For this review, take the finished solid that the model builds, in its own axes (mm). Face numbers are marked on the shaded views. A direction names the side the tool comes from. Round coordinates to 2 decimals unless told otherwise and drop trailing zeros. Write each loop counter-clockwise with the first axis right and the second up, starting at its lowest first coordinate (ties: lowest second). Pieces come first, ordered by that corner, then holes. Notation, with made-up numbers: M -18,-12.75 L -11,-12.75 A27 cw -11,19.25 Z; hole C 53,20 d9. An arc over 180 degrees is marked long. Write each question's results on one line, items separated by ' | '. Start each with the question number.
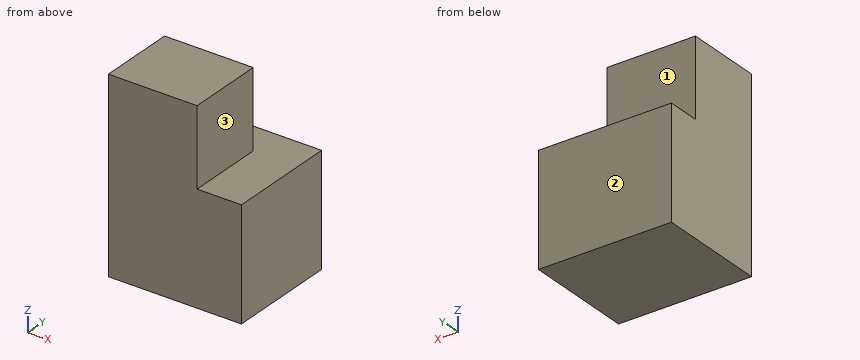
```python
from build123d import *

# Parameters (mm, degrees)
F1_W     = 40
F1_H     = 35
F3_DEPTH = 50
F2_W     = 40
F2_H     = 35
F4_DEPTH = 35


with BuildPart() as f3:
    # F1 (on Top) → F3 (new body)
    with BuildSketch(Plane.XY):
        with Locations((-10, -7.5)):
            Rectangle(F1_W, F1_H)
        Polygon((30, 25), (-30, 25), (-30, 10), (10, 10), (10, -25), (30, -25), align=None)
    extrude(amount=F3_DEPTH)

    # F2 (on offset) → F4 (join)
    with BuildSketch(Plane.XY.offset(50)):
        with Locations((-10, -7.5)):
            Rectangle(F2_W, F2_H)
    extrude(amount=F4_DEPTH)


solid = f3.part
```
Item 1: For probe 1 along Z at (x, y) = (-10.5, 17.5); probe 2 along Y at (x, z) = (6, 79.5); probe 3 along X at (y, z) = (-6.5, 65), list the stretches that pass through material, from the lowest coordinate up.
Item 2: For the marked faces 1, 2 and 3, list the 3-axis set-ups (+Z, -Z, +X, -X, +Y, -Y) from which the entire face can be reached by the end or side of a thin tool; tool diameter is ignored.
Item 3: We need section B-B on y = -19.5. State the section outline as (x, z) points, then the cut area to 3 significant figures.
Item 4: We need section A-A on x = -2. State the section outline as (y, z) points, then the cut area to 4 significant figures.
Item 5: We need section D-D on y = 15. State the section outline as (x, z) points, then the cut area to 3 significant figures.
Item 6: Insertion check: P1, Ø4, axis at x = -16.5, z = 75.5, coming from the +Y side. The pin has a flat end and moves straight along its axis. Give the tip position at first contact, or say it passes through.
Item 7: We need section C-C on z = 64. State the section outline as (x, y) points, then the cut area to 3 significant figures.
Numbers:
1) probe 1: z = 0 to 50 | probe 2: y = -25 to 10 | probe 3: x = -30 to 10
2) face 1: +Z, +X, -X, +Y | face 2: +Z, -Z, +X, -X, +Y | face 3: +Z, +X, +Y, -Y
3) outline: M -30,0 L 30,0 L 30,50 L 10,50 L 10,85 L -30,85 Z | area: 4,400 mm^2
4) outline: M -25,0 L 25,0 L 25,50 L 10,50 L 10,85 L -25,85 Z | area: 3,725 mm^2
5) outline: M -30,0 L 30,0 L 30,50 L -30,50 Z | area: 3,000 mm^2
6) P1: stops at y = 10
7) outline: M -30,-25 L 10,-25 L 10,10 L -30,10 Z | area: 1,400 mm^2
